The model under review builds one solid part; all positions refer to its coordinate system, in mm. Face numbers are marked on the shaded views. A direction names the side the tool comes from. Give positions to 0.01 mm unless a question says otherwise; leave off trailing zeros. Loops run counter-clockwise (first coordinate to the right, second up) from the corner with the lowest first, then second, coordinate; pieces in that order, holes last. Notation, with made-up numbers: M 48,-35.75 L 53,-35.75 A25 cw 53,-18.75 Z; hole C 61.5,36 d7. An arc over 180 degrees is marked long. One line per item, written item: value. Start each with the question number.
Q1. We need section B-B on y = 17.5. Write out the cut boundary in (x, z).
Q2. Mouldability with a two-part tool opening along X and no side actions: class the marked faces 3, 4 and 5 as released by +X, released by -X, zero draft, split by the parting line, or undercut.
Q3. For the marked faces 1 and 2, list the 3-axis set-ups (+Z, -Z, +X, -X, +Y, -Y) from which the entire face can be reached by the end or side of a thin tool; tool diameter is ignored.
Q4. We need section C-C on x = 30. Write out the cut boundary in (y, z).
Q5. We need section D-D on z = 5.5. Write out the cut boundary in (x, y), plus the area to 3 significant figures.
Q6. We need section A-A on z = 13.4. Give the number of separate pieces and of enclosed holes in the cut face, plus the area to 3 significant figures.
Q7. For pin 1 (5.5 mm diameter, centred on y = 17.5, z = 13.4, fed in from +X); pin 2 (1.5 mm diameter, centred on x = 34.5, z = 17, fed in from +Y); pin 3 (5 mm diameter, centred on x = 28.5, y = -5, fed in from +Z); pin 4 (1 mm diameter, centred on x = 14, z = 11, fed in from -Y), all flat-tipped, find the tip position at first contact; note any pin that passes through.
Q8. To check wall thickness, follow line 1 along Y through (x, z) = (30, 6.75); line 2 along X through (y, z) = (17, 2.5); line 3 along Y through (x, z) = (53, 7.25). State the ranges of each line that lie inside material, in increasing order. Write a range as from..to.
```python
from build123d import *

# Parameters (mm, degrees)
F0_W     = 60
F0_H     = 35
F1_DEPTH = 1.8
F3_DEPTH = 25
F0_R     = 2
F4_DEPTH = 15
F5_R     = 3.5
F6_DEPTH = 63.601


with BuildPart() as f1:
    # F0 (on Top) → F1 (new body)
    with BuildSketch(Plane.XY):
        Polygon((26, 36.8), (-1.8, 36.8), (-1.8, -1.8), (26, -1.8), (34, -1.8), (61.8, -1.8), (61.8, 36.8), (34, 36.8), align=None)
        with Locations((30, 17.5)):
            Rectangle(F0_W, F0_H, mode=Mode.SUBTRACT)
        with Locations((30, 17.5)):
            Rectangle(F0_W, F0_H)
    extrude(amount=F1_DEPTH)

    # F2 (on face) → F3 (join)
    with BuildSketch(Plane.XY.offset(1.8)):
        Polygon((-1.8, -1.8), (15.426563, -1.8), (61.8, -1.8), (61.8, 36.8), (-1.8, 36.8), align=None)
        Polygon((16.889177, 0), (0, 0), (0, 35), (60, 35), (60, 0), align=None, mode=Mode.SUBTRACT)
    extrude(amount=F3_DEPTH)

    # F0 (on Top) → F4 (join)
    with BuildSketch(Plane.XY):
        with BuildLine():
            Line((34, -1.8), (26, -1.8))
            Line((26, -1.8), (26, -4.8))
            ThreePointArc((26, -4.8), (26.87868, -6.92132), (29, -7.8))
            Line((29, -7.8), (31, -7.8))
            ThreePointArc((31, -7.8), (33.12132, -6.92132), (34, -4.8))
            Line((34, -4.8), (34, -1.8))
        make_face()
        with Locations((30, -4.8)):
            Circle(F0_R, mode=Mode.SUBTRACT)
        with BuildLine():
            Line((26, 39.8), (26, 36.8))
            Line((26, 36.8), (34, 36.8))
            Line((34, 36.8), (34, 39.8))
            ThreePointArc((34, 39.8), (33.12132, 41.92132), (31, 42.8))
            Line((31, 42.8), (29, 42.8))
            ThreePointArc((29, 42.8), (26.87868, 41.92132), (26, 39.8))
        make_face()
        with Locations((30, 39.8)):
            Circle(F0_R, mode=Mode.SUBTRACT)
    extrude(amount=F4_DEPTH)

    # F5 (on face) → F6 (cut, through all)
    with BuildSketch(Plane.YZ.offset(61.8)):
        with Locations((17.5, 13.4)):
            Circle(F5_R)
    extrude(amount=-F6_DEPTH, mode=Mode.SUBTRACT)


solid = f1.part
```
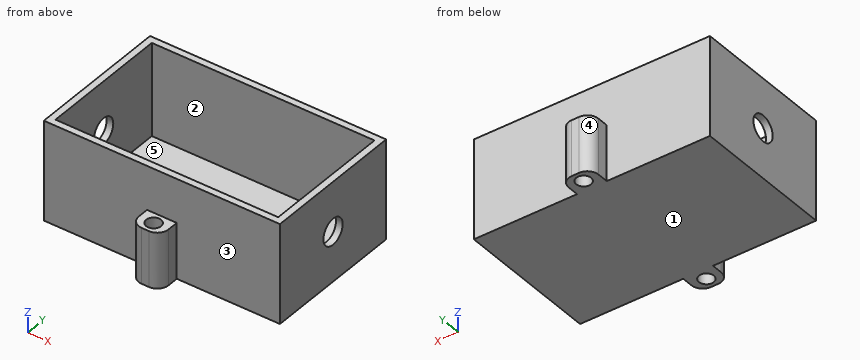
Solved:
1. outline: M -1.8,0 L 61.8,0 L 61.8,9.9 L 60,9.9 L 60,1.8 L 0,1.8 L 0,9.9 L -1.8,9.9 Z; M -1.8,16.9 L 0,16.9 L 0,26.8 L -1.8,26.8 Z; M 60,16.9 L 61.8,16.9 L 61.8,26.8 L 60,26.8 Z
2. face 3: zero draft
2. face 4: released by -X
2. face 5: undercut
3. face 1: -Z, +X, -X, +Y, -Y
3. face 2: +Z
4. outline: M -7.8,0 L -6.8,0 L -6.8,15 L -7.8,15 Z; M -2.8,0 L 37.8,0 L 37.8,15 L 36.8,15 L 36.8,26.8 L 35,26.8 L 35,1.8 L 0,1.8 L 0,26.8 L -1.8,26.8 L -1.8,15 L -2.8,15 Z; M 41.8,0 L 42.8,0 L 42.8,15 L 41.8,15 Z
5. outline: M -1.8,-1.8 L 26,-1.8 L 26,-4.8 A3 ccw 29,-7.8 L 31,-7.8 A3 ccw 34,-4.8 L 34,-1.8 L 61.8,-1.8 L 61.8,36.8 L 34,36.8 L 34,39.8 A3 ccw 31,42.8 L 29,42.8 A3 ccw 26,39.8 L 26,36.8 L -1.8,36.8 Z; hole M 0,0 L 60,0 L 60,35 L 0,35 Z; hole C 30,-4.8 d4; hole C 30,39.8 d4
5. area: 418 mm2
6. separate pieces: 2
6. enclosed holes: 2
6. area: 393 mm2
7. pin 1: through
7. pin 2: y = 36.8
7. pin 3: z = 15
7. pin 4: y = -1.8
8. line 1: -7.8..-6.8, -2.8..0, 35..37.8, 41.8..42.8
8. line 2: -1.8..0, 60..61.8
8. line 3: -1.8..0, 35..36.8
